The listing builds one solid part. Answer for the finished solid, in the listing's coordinates (mm). A direction names the side the tool comes from. Round coordinates to 2 decimals unless told otherwise and drop trailing zeros. Order: outer loops, then holes, each group sorted by start corner. A loop starts at its lowest first (then second) coordinate and runs counter-clockwise, first axis right, second up. Notation, with made-up numbers: (-1, 10) - (56, 10) arc R18 ccw to (56, 23) - close; hole circle Ø1 at (-27.75, 40). An arc over 180 degrees is marked (long way). Use CSV: the item, a comma, the result in double quotes. Start each with the question number.
Item 1: Determine the mould class of faces 1 (the cylindrical face through (52.126, 1002.786, 24.458)), 2 (the flat face through (495, 1014, -21.5)), 3 (the flat face through (507, 2000, 0)) for opening direction Y: +Y half, -Y half, draft (parallel to the pull), parting line (faces both ways), or undercut.
Item 2: Find section A-A, the plane y = 900. Give the vertices of the cut face in (x, z).
Item 3: Flat-ended cylindrical pins translate along their axes: P1, Ø1.2, axis at x = 1.5, y = 949, coming from the -Z side; P2, Ø4.5, axis at x = 2, y = 599.5, coming from the +Z side; P3, Ø2, axis at y = 762, z = 20, coming from the -X side; P4, Ø11.5, axis at x = 56.5, y = 1028.7, coming from the +Z side. Find the tip coordinate at first contact, or state that the pin passes through.
Item 4: For faces 4 (the cylindrical face through (49.455, 931.727, 24.458)), 5 (the flat face through (0, 1014, 0)), determine the directions among +Z, -Z, +X, -X, +Y, -Y from which every point of the face is accessible in a straight line to the end or side of a thin tool.
Item 5: Find section B-B, the plane x = 493. Give the vertices of the cut face in (y, z), plus the area to 3 significant figures.
Item 6: Find section C-C, the plane y = 1688. Give the vertices of the cut face in (x, z), plus the area to 3 significant figures.
Item 7: Straight lines are drawn through the part: line 1 along Y through (x, z) = (56.5, 23.85); line 2 along X through (y, z) = (1028.7, 23.55) (3 decimals); line 3 along Z through (x, y) = (350.5, 460.5). For each, find the intervals that lie inside material, in ascending order. Write a range as [from, to].
Autodesk Inventor part; units mm, degrees
ref_plane "YZ Plane" through (0, 0, 0) normal (1, 0, 0) x (0, 1, 0)
ref_plane "XZ Plane" through (0, 0, 0) normal (0, 1, 0) x (-1, 0, 0)
ref_plane "XY Plane" through (0, 0, 0) normal (0, 0, 1) x (1, 0, 0)
sketch "Sketch1" plane through (0, 0, 0) normal (0, 0, 1) x (1, 0, 0)
  line L0 (0, 0) -> (1000, 0)
  line L1 (1000, 0) -> (1000, 2000)
  line L2 (1000, 2000) -> (0, 2000)
  line L3 (0, 2000) -> (0, 0)
  line L4 (0, 0) -> (4, 0)
  line L5 (0, 0) -> (4, 0) construction
  line L6 (4, 0) -> (4, 2000)
  line L7 (4, 0) -> (4, 900)
  line L8 (4, 900) -> (24, 900)
  line L9 (24, 900) -> (56.5, 900)
  circle A0 centre (56.5, 900) radius 32.5
  line L10 (56.5, 932.5) -> (56.5, 1002.5)
  line L11 (56.5, 1002.5) -> (56.5, 1036.1)
  circle A1 centre (56.5, 1036.1) radius 33.6
  line L12 (56.5, 1069.7) -> (56.5, 1037.7)
  line L13 (56.5, 1037.7) -> (56.5, 1064.7)
  line L14 (56.5, 1064.7) -> (56.5, 1028.7)
  line L15 (56.5, 1028.7) -> (56.5, 1010.7)
  line L16 (56.5, 1010.7) -> (58.505, 1010.7)
  line L17 (56.5, 1064.7) -> (58.505, 1064.7)
  line L18 (60.4989, 1062.8571) -> (63.008, 1031.0205)
  line L19 (60.478, 1012.372) -> (62.8086, 1026.3917)
  arc A2 (62.8086, 1026.3917) -> (63.008, 1031.0205) centre (43.9839, 1029.5211) ccw
  arc A3 (60.4989, 1062.8571) -> (58.505, 1064.7) centre (58.505, 1062.7) ccw
  arc A4 (58.505, 1010.7) -> (60.478, 1012.372) centre (58.505, 1012.7) ccw
  line L20 (63.0493, 1028.7) -> (56.5, 1028.7)
  circle A5 centre (56.5, 1028.7) radius 5
  point P0 (60.2, 1010.7)
  point P1 (60.3536, 1064.7)
  point P2 (49.8, 1028.7)
  dimension "d11" = 65
  dimension "d0" = 1000
  dimension "d1" = 2000
  dimension "d2" = 4
  dimension "d8" = 900
  dimension "d9" = 20
  dimension "d10" = 32.5
  dimension "d12" = 70
  dimension "d13" = 33.6
  dimension "d24" = 32
  dimension "d25" = 27
  dimension "d26" = 36
  dimension "d27" = 18
  dimension "d28" = 3.7
  dimension "d31" = 2
  dimension "d32" = 6.5493
  dimension "d33" = 10
extrude "Extrusion1" add sketch "Sketch1" along normal mid plane 43 contours A1 L12 L14 L11 A5 | L11 L16 A4 L19 A2 L18 A3 L17 L12 A1 | A0 | L6 L2 L1 L0 | L11 A5 L20 A2 L19 A4 L16 | A5 L11 | L11 L20 A5 | L17 A3 L18 A2 L20 A5 L11 L14 L12 | L11 A5 L20
extrude "Extrusion2" add sketch "Sketch1" along normal mid plane 35 contours L3 L2 L6 L0
extrude "Extrusion3" add sketch "Sketch1" along normal blind 6 from surface at 21.5 contours A1 L12 L14 L11 A5 | L11 L16 A4 L19 A2 L18 A3 L17 L12 A1 | A0 | L11 A5 L20 A2 L19 A4 L16 | A5 L11 | L11 L20 A5 | L17 A3 L18 A2 L20 A5 L11 L14 L12 | L11 A5 L20
sketch "Sketch2" plane through (0, 0, 17.5) normal (-1, 0, 0) x (0, 0, 1)
  line L0 (-35, 0) -> (-35, 2000)
  line L1 (-17.5, 0) -> (1182.5, 0) construction
  line L2 (10, 1069.7) -> (10, 1002.5)
  line L3 (10, 1036.1) -> (-17.5, 1036.1)
  line L4 (10, 932.5) -> (10, 867.5)
  line L5 (10, 900) -> (-17.5, 900)
  line L6 (-27.5, 877.5) -> (-7.5, 877.5)
  line L7 (-7.5, 877.5) -> (-7.5, 922.5)
  line L8 (-7.5, 922.5) -> (-27.5, 922.5)
  line L9 (-27.5, 922.5) -> (-27.5, 877.5)
  line L10 (-27.5, 877.5) -> (-7.5, 922.5) construction
  line L11 (-7.5, 877.5) -> (-27.5, 922.5) construction
  line L12 (-17.5, 0) -> (-17.5, 2000)
  line L13 (10, 932.5) -> (-17.5, 932.5)
  line L14 (-27.5, 1011.1) -> (-7.5, 1011.1)
  line L15 (-7.5, 1011.1) -> (-7.5, 1061.1)
  line L16 (-7.5, 1061.1) -> (-27.5, 1061.1)
  line L17 (-27.5, 1061.1) -> (-27.5, 1011.1)
  line L18 (-27.5, 1011.1) -> (-7.5, 1061.1) construction
  line L19 (-7.5, 1011.1) -> (-27.5, 1061.1) construction
  dimension "d20" = 20
  dimension "d21" = 45
  dimension "d22" = 20
  dimension "d23" = 50
extrude "Extrusion4" cut sketch "Sketch1" against normal blind 6 from surface at 27.5 contours A5 L11 | L11 L20 A5 | L11 A5 L20
properties part number "door"
Worked out:
1,face 1,"undercut"
1,face 2,"draft"
1,face 3,"+Y half"
2,outline,"(0, -17.5) - (4, -17.5) - (4, -21.5) - (1000, -21.5) - (1000, 21.5) - (89, 21.5) - (89, 27.5) - (24, 27.5) - (24, 21.5) - (4, 21.5) - (4, 17.5) - (0, 17.5) - close"
3,P1,"stops at z = -17.5"
3,P2,"stops at z = 21.5"
3,P3,"stops at x = 4"
3,P4,"stops at z = 27.5"
4,face 4,"+Z"
4,face 5,"+Z, -Z, -X, +Y, -Y"
5,outline,"(0, -21.5) - (2000, -21.5) - (2000, 21.5) - (0, 21.5) - close"
5,area,"86,000 mm²"
6,outline,"(0, -17.5) - (4, -17.5) - (4, -21.5) - (1000, -21.5) - (1000, 21.5) - (4, 21.5) - (4, 17.5) - (0, 17.5) - close"
6,area,"43,000 mm²"
7,line 1,"y = [867.5, 932.5], [1002.5, 1023.7], [1033.7, 1069.7]"
7,line 2,"x = [23.725, 51.5], [61.5, 89.275]"
7,line 3,"z = [-21.5, 21.5]"
